Input: dimensioned drawing with shaded views. Units: mm. Origin: part minimum x, y, z. Round coordinates to 2 decimals unless told otherwise and drop trailing zeros. Loops run counter-clockwise (first coordinate to the right, second up) from the corner with the lowest first, then second, coordinate; pieces in that order, holes last. Notation, with made-up numbers: (36.5, 70) - (48.5, 70) arc R27 cw to (48.5, 102) - close; hole circle Ø6 at (82, -33). An arc over 180 degrees is marked (long way). Answer as CSV lines item,"result".
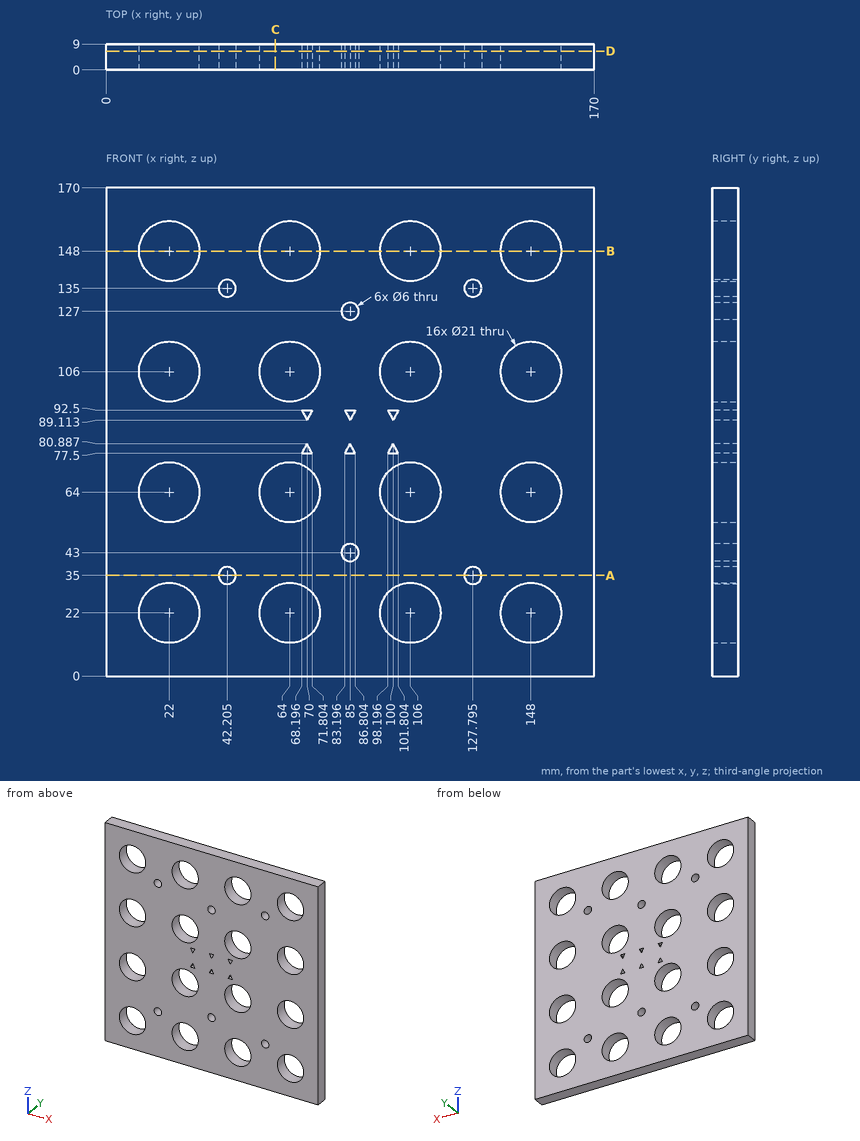
(1) Section A-A (z = 35). Output: boundary loops of the cut face in (x, y) (1 decimal).
Findings below:
outline,"(0, 0) - (39.2, 0) - (39.2, 9) - (0, 9) - close; (45.2, 0) - (124.8, 0) - (124.8, 9) - (45.2, 9) - close; (130.8, 0) - (170, 0) - (170, 9) - (130.8, 9) - close"
(2) Section B-B (z = 148). Output: boundary loops of the cut face in (x, y).
Findings below:
outline,"(0, 0) - (11.5, 0) - (11.5, 9) - (0, 9) - close; (32.5, 0) - (53.5, 0) - (53.5, 9) - (32.5, 9) - close; (74.5, 0) - (95.5, 0) - (95.5, 9) - (74.5, 9) - close; (116.5, 0) - (137.5, 0) - (137.5, 9) - (116.5, 9) - close; (158.5, 0) - (170, 0) - (170, 9) - (158.5, 9) - close"
(3) Section C-C (x = 59). Output: boundary loops of the cut face in (y, z).
Findings below:
outline,"(0, 0) - (9, 0) - (9, 12.77) - (0, 12.77) - close; (0, 31.23) - (9, 31.23) - (9, 54.77) - (0, 54.77) - close; (0, 73.23) - (9, 73.23) - (9, 96.77) - (0, 96.77) - close; (0, 115.23) - (9, 115.23) - (9, 138.77) - (0, 138.77) - close; (0, 157.23) - (9, 157.23) - (9, 170) - (0, 170) - close"
(4) Material intervals for line 1 along X through (y, z) = (4.75, 64); line 2 along X through (y, z) = (2.25, 135) (1 decimal), sorted ascending.
Findings below:
line 1,"0 to 11.5, 32.5 to 53.5, 74.5 to 95.5, 116.5 to 137.5, 158.5 to 170"
line 2,"0 to 39.2, 45.2 to 124.8, 130.8 to 170"
(5) Section D-D (y = 6.5). Give the number of separate pieces and of enclosed holes in the cut face, and give its area (3 significant figures).
Findings below:
separate pieces,"1"
enclosed holes,"28"
area,"23,200 mm2"
